Source: three-view drawing plus pictorial views. Frame: mm from the lowest corner of the part. A direction names the side the tool comes from. Give positions to 0.01 mm unless a question says otherwise; leave off trailing zeros. Loops run counter-clockwise (first coordinate to the right, second up) from the corner with the lowest first, then second, coordinate; pieces in that order, holes last. Notation, with made-up numbers: (-10, 78.25) - (21, 78.25) arc R12 ccw to (21, 94.25) - close; hole circle Ø5 at (59, 20). An arc over 180 degrees is marked (long way). Answer as a JSON object with one key per item and string values.
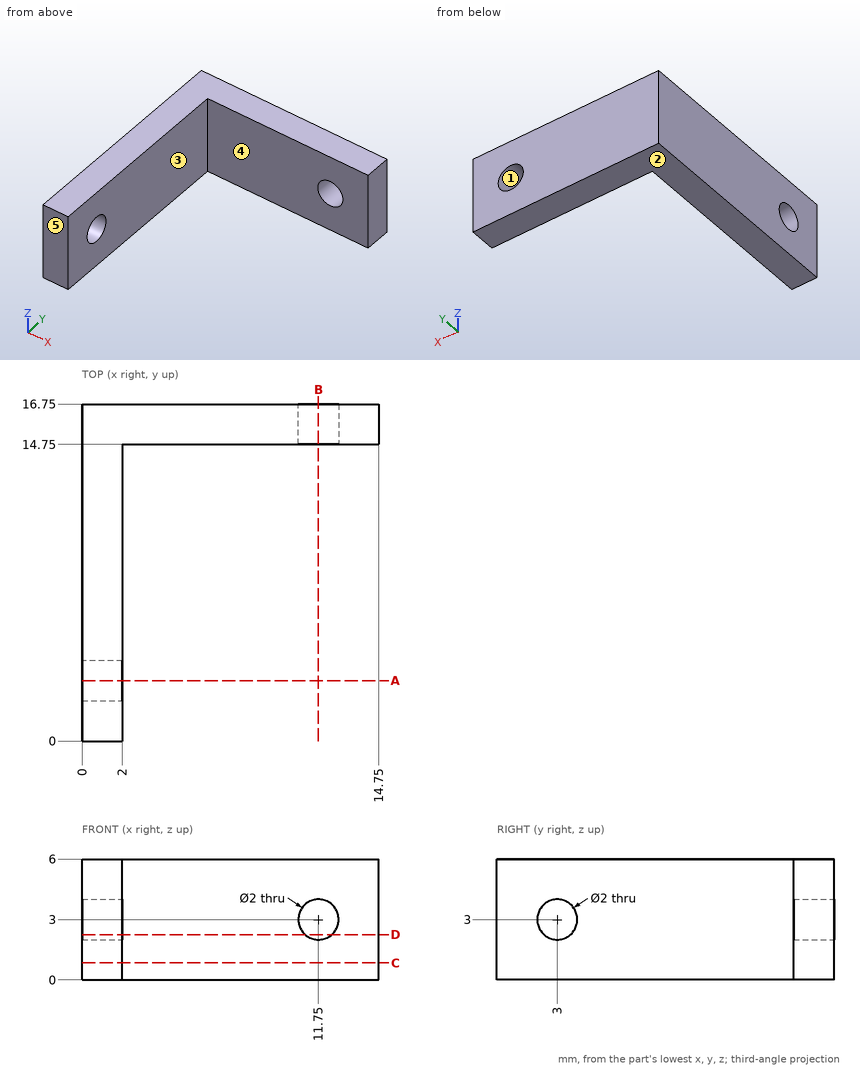
Item 1: Material intervals for line 1 (Z direction, x = 1.5, y = 3); line 2 (X direction, y = 14.5, z = 1.75); line 3 (Y direction, x = 8.5, z = 5.7), sorted ascending. Write a range as [from, to].
Geometry check:
{"line 1": "z = [0, 2], [4, 6]", "line 2": "x = [0, 2]", "line 3": "y = [14.75, 16.75]"}
Item 2: Cut plane D-D (z = 2.25). Return loops of the section in (x, y), then the cut area to 3 significant figures.
Geometry check:
{"outline": "(0, 0) - (2, 0) - (2, 2.34) - (0, 2.34) - close; (0, 3.66) - (2, 3.66) - (2, 14.75) - (11.09, 14.75) - (11.09, 16.75) - (0, 16.75) - close; (12.41, 14.75) - (14.75, 14.75) - (14.75, 16.75) - (12.41, 16.75) - close", "area": "53.7 mm2"}
Item 3: Cut plane B-B (x = 11.75). Return loops of the section in (y, z), then the cut area to 3 significant figures.
Geometry check:
{"outline": "(14.75, 0) - (16.75, 0) - (16.75, 2) - (14.75, 2) - close; (14.75, 4) - (16.75, 4) - (16.75, 6) - (14.75, 6) - close", "area": "8.00 mm2"}
Item 4: Mould query, pull axis Z, two halves, no side actions, for the marked faces 1, 2 and 3. Classes: released by +Z, released by -Z, zero draft, split by the parting line, or undercut.
Geometry check:
{"face 1": "undercut", "face 2": "released by -Z", "face 3": "zero draft"}
Item 5: Cut plane C-C (z = 0.85). Return loops of the section in (x, y).
Geometry check:
{"outline": "(0, 0) - (2, 0) - (2, 14.75) - (14.75, 14.75) - (14.75, 16.75) - (0, 16.75) - close"}
Item 6: Cut plane A-A (y = 3). Return loops of the section in (x, z), then the cut area to 3 significant figures.
Geometry check:
{"outline": "(0, 0) - (2, 0) - (2, 2) - (0, 2) - close; (0, 4) - (2, 4) - (2, 6) - (0, 6) - close", "area": "8.00 mm2"}
Item 7: Access query for the marked faces 4 and 5. Directions: +Z, -Z, +X, -X, +Y, -Y. A direction counts if a zero-diameter tool reaches every point of the face in a straight line with its end or side. Return the directions, or none.
Geometry check:
{"face 4": "+Z, -Z, +X, -Y", "face 5": "+Z, -Z, +X, -X, -Y"}
Item 8: Contact query for flat-ended pins moving along their axis: P1, Ø3, axis at y = 6, z = 1.5, coming from the +X side; P2, Ø3, axis at x = 6, z = 4.5, coming from the -Y side. Output: stop coordinate, or through.
Geometry check:
{"P1": "stops at x = 2", "P2": "stops at y = 14.75"}
